from build123d import *

# Parameters (mm, degrees)
SKETCH1_W            = 66.04
SKETCH1_H            = 43.815
BOSS_EXTRUDE1_DEPTH  = 3.175
M3_CLEARANCE_HOLE1_D = 3.4
SKETCH6_W            = 22.86
SKETCH6_H            = 9.652
CUT_EXTRUDE1_DEPTH   = 4.175
FILLET1_R            = 0.508
FILLET2_R            = 2.54
SKETCH7_W            = 12.7
SKETCH7_H            = 66.04
BOSS_EXTRUDE2_DEPTH  = 3.175
M3_CLEARANCE_HOLE2_D = 3.4
FILLET3_R            = 2.54
CUT_EXTRUDE2_DEPTH   = 4.175


with BuildPart() as part:
    # Sketch1 → Boss-Extrude1 (new body)
    with BuildSketch(Plane(origin=(0, 0, 0), x_dir=(1, 0, 0), z_dir=(0, 1, 0))):
        with Locations((33.02, 21.9075)):
            Rectangle(SKETCH1_W, SKETCH1_H)
    extrude(amount=BOSS_EXTRUDE1_DEPTH)

    # M3 Clearance Hole1 (through all)
    with Locations(Plane(origin=(0, 0, 0), x_dir=(-1, 0, 0), z_dir=(0, -1, 0))):
        with Locations((-5.08, 6.858), (-5.08, 36.957), (-48.1203, 36.957), (-48.1203, 6.858), (-60.96, 6.858), (-60.96, 36.957)):
            Hole(M3_CLEARANCE_HOLE1_D / 2)

    # Sketch6 → Cut-Extrude1 (cut, through all)
    with BuildSketch(Plane(origin=(0, 3.175, 0), x_dir=(1, 0, 0), z_dir=(0, 1, 0))):
        with Locations((33.3248, 26.289)):
            Rectangle(SKETCH6_W, SKETCH6_H)
    extrude(amount=-CUT_EXTRUDE1_DEPTH, mode=Mode.SUBTRACT)

    # Fillet1
    fillet1_edges = [part.edges().sort_by_distance(p)[0] for p in [
        (44.7548, 1.5875, -21.463),
        (21.8948, 1.5875, -21.463),
        (21.8948, 1.5875, -31.115),
        (44.7548, 1.5875, -31.115),
    ]]
    fillet(fillet1_edges, radius=FILLET1_R)

    # Fillet2
    fillet2_edges = [part.edges().sort_by_distance(p)[0] for p in [
        (0, 1.5875, -43.815),
        (66.04, 1.5875, -43.815),
        (66.04, 1.5875, 0),
        (0, 1.5875, 0),
    ]]
    fillet(fillet2_edges, radius=FILLET2_R)

    # Sketch7 → Boss-Extrude2 (add)
    with BuildSketch(Plane(origin=(0, 3.175, 0), x_dir=(1, 0, 0), z_dir=(0, 1, 0))):
        with Locations((59.69, 21.9075)):
            Rectangle(SKETCH7_W, SKETCH7_H)
    extrude(amount=-BOSS_EXTRUDE2_DEPTH)

    # M3 Clearance Hole2 (through all)
    with Locations(Plane(origin=(0, 3.175, 0), x_dir=(1, 0, 0), z_dir=(0, 1, 0))):
        with Locations((60.96, 49.8475), (60.96, -6.0325)):
            Hole(M3_CLEARANCE_HOLE2_D / 2)

    # Fillet3
    fillet3_edges = [part.edges().sort_by_distance(p)[0] for p in [
        (53.34, 1.5875, 11.1125),
        (66.04, 1.5875, -54.9275),
        (53.34, 1.5875, -54.9275),
        (53.34, 1.5875, 0),
        (53.34, 1.5875, -43.815),
        (66.04, 1.5875, 11.1125),
    ]]
    fillet(fillet3_edges, radius=FILLET3_R)

    # Sketch11 → Cut-Extrude2 (cut, through all)
    with BuildSketch(Plane.XZ):
        with BuildLine():
            Line((3.38, -6.858), (3.38, -7.62))
            ThreePointArc((3.38, -7.62), (5.08, -9.32), (6.78, -7.62))
            Line((6.78, -7.62), (6.78, -6.858))
            ThreePointArc((6.78, -6.858), (5.08, -5.158), (3.38, -6.858))
        make_face()
        with BuildLine():
            Line((6.78, -36.195), (6.78, -36.957))
            ThreePointArc((6.78, -36.957), (5.08, -38.657), (3.38, -36.957))
            Line((3.38, -36.957), (3.38, -36.195))
            ThreePointArc((3.38, -36.195), (5.08, -34.495), (6.78, -36.195))
        make_face()
    extrude(amount=-CUT_EXTRUDE2_DEPTH, mode=Mode.SUBTRACT)


solid = part.part
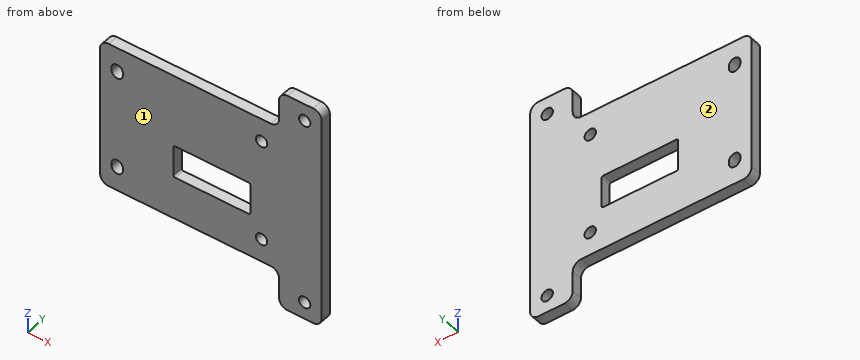
Design review of the part built by this model. Coordinates are the model's own, in mm. Face numbers are marked on the shaded views. Give positions to 0.01 mm unless a question says otherwise; leave off trailing zeros. Write each loop counter-clockwise with the first axis right and the second up, starting at its lowest first coordinate (ties: lowest second). Pieces come first, ordered by that corner, then holes. Notation, with made-up numbers: M -20.5,18 L -7.5,18 A20 ccw -7.5,49 Z; hole C -8,-2.75 d9. An arc over 180 degrees is marked long. Return JSON: item names as keys, results as strings. Group by question number.
Item 1: Clearance check with flat-ended pins moving along their axes: pin 1 Ø10 at (x, z) = (17.5, -41) entering from -Y; pin 2 Ø1 at (y, z) = (2, -48) entering from -X; pin 3 Ø1 at (y, z) = (3, -45.5) entering from -X. State where each tip first meets the part, or that it passes through.
Item 2: Take a section at C-C (x = 34.5). Give the boundary of the cut face in (y, z) (3 decimals), plus the area to 3 significant figures.
Item 3: Take a section at A-A (x = 60.96). Give the boundary of the cut face in (y, z) (1 decimal).
Item 4: Take a section at B-B (z = -29). Give the boundary of the cut face in (x, y) (3 decimals).
Item 5: The part is to be moulded in two halves that separate along Y. For the marked faces 1 and 2, say which applies: pulls with the +Y half, pulls with the -Y half, needs draft (parallel to the pull), parting line crosses it, or undercut.
Item 6: Take a section at D-D (x = 5.08). Give the boundary of the cut face in (y, z) (3 decimals).
Item 7: Wall thickness on line 1 along Z through (x, y) = (60.96, 2.5); line 2 along Z through (x, y) = (6.5, 1.05) (3 decimals); line 3 along Z through (x, y) = (34, 1.55) (3 decimals): over which ranges is each line inside the solid? List them lowest first.
Return value:
{
 "1": {"pin 1": "stops at y = 0", "pin 2": "stops at x = 53.34", "pin 3": "stops at x = 52.95"},
 "2": {"outline": "M 0,-43.815 L 3.175,-43.815 L 3.175,-31.115 L 0,-31.115 Z; M 0,-21.463 L 3.175,-21.463 L 3.175,0 L 0,0 Z", "area": "108 mm2"},
 "3": {"outline": "M 0,-54.9 L 3.2,-54.9 L 3.2,-51.5 L 0,-51.5 Z; M 0,-48.1 L 3.2,-48.1 L 3.2,4.3 L 0,4.3 Z; M 0,7.7 L 3.2,7.7 L 3.2,11.1 L 0,11.1 Z"},
 "4": {"outline": "M 0,0 L 21.895,0 L 21.895,3.175 L 0,3.175 Z; M 44.755,0 L 66.04,0 L 66.04,3.175 L 44.755,3.175 Z"},
 "5": {"face 1": "pulls with the -Y half", "face 2": "pulls with the +Y half"},
 "6": {"outline": "M 0,-43.815 L 3.175,-43.815 L 3.175,-38.657 L 0,-38.657 Z; M 0,-34.495 L 3.175,-34.495 L 3.175,-9.32 L 0,-9.32 Z; M 0,-5.158 L 3.175,-5.158 L 3.175,0 L 0,0 Z"},
 "7": {"line 1": "z = -54.93 to -51.55, -48.15 to 4.33, 7.73 to 11.11", "line 2": "z = -43.815 to -37.892, -35.26 to -8.555, -5.923 to 0", "line 3": "z = -43.815 to -31.115, -21.463 to 0"}
}
